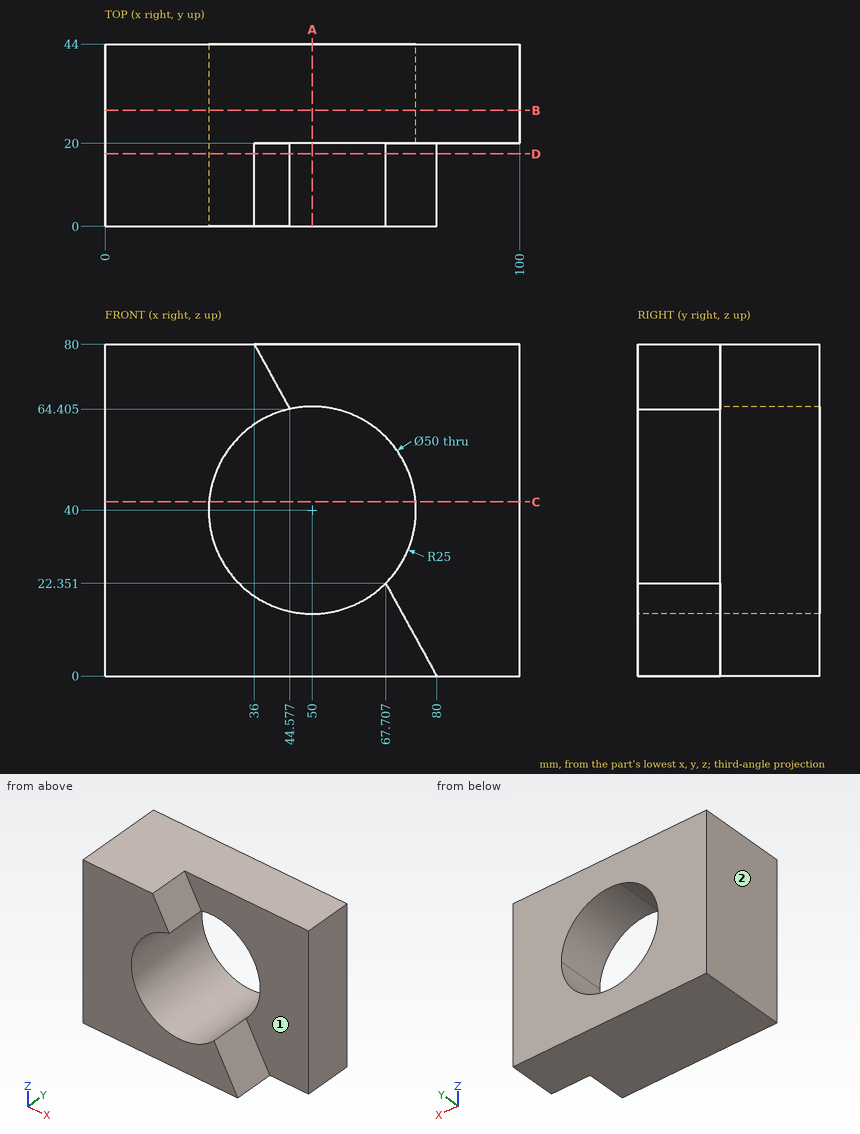
The figure shows three views and two pictorial views of one solid part (mm, origin at its lowest corner). Answer the questions. A direction names the side the tool comes from. Coordinates: 2 decimals unless noted, no trailing zeros. Write each loop counter-clockwise with the first axis right and the second up, starting at its lowest first coordinate (ties: lowest second). Pieces come first, ordered by that corner, then holes.
1. The part is cut by section B-B, the plane y = 28. Write down the section's boundary in (x, z) (1 decimal).
Results list:
outline: (0, 0) - (100, 0) - (100, 80) - (0, 80) - close; hole (67.7, 22.4) arc R25 ccw to (75, 40) arc R25 ccw (long way) to start
2. The part is cut by section A-A, the plane x = 50. Write down the section's boundary in (y, z), and give its area (3 significant figures).
Results list:
outline: (0, 0) - (44, 0) - (44, 15) - (0, 15) - close; (20, 65) - (44, 65) - (44, 80) - (20, 80) - close
area: 1,020 mm2
3. Consider line 1 along X through (y, z) = (28.5, 40); line 2 along Y through (x, z) = (91, 27); line 3 along Z through (x, y) = (50.5, 31.5) (1 decimal). Determine where each line is inside the solid, lowest interval first.
Results list:
line 1: x = 0 to 25, 75 to 100
line 2: y = 20 to 44
line 3: z = 0 to 15, 65 to 80
4. For the marked faces 1 and 2, determine the directions among +Z, -Z, +X, -X, +Y, -Y from which every point of the face is accessible in a straight line to the end or side of a thin tool.
Results list:
face 1: +Z, +X, -Y
face 2: +Z, -Z, -X, +Y, -Y
5. The part is cut by section D-D, the plane y = 17.5. Write down the section's boundary in (x, z) (1 decimal), and give its area (3 significant figures).
Results list:
outline: (0, 0) - (80, 0) - (67.7, 22.4) arc R25 cw (long way) to (44.6, 64.4) - (36, 80) - (0, 80) - close
area: 3,310 mm2
6. The part is cut by section C-C, the plane z = 42. Write down the section's boundary in (x, y), and give its area (3 significant figures).
Results list:
outline: (0, 0) - (25.08, 0) - (25.08, 44) - (0, 44) - close; (74.92, 20) - (100, 20) - (100, 44) - (74.92, 44) - close
area: 1,710 mm2
